The model under review builds one solid part; all positions refer to its coordinate system, in mm. A direction names the side the tool comes from. Round coordinates to 2 decimals unless told otherwise and drop trailing zeros. Write each loop counter-clockwise with the first axis right and the second up, starting at its lowest first coordinate (ties: lowest second). Pieces come first, ordered by that corner, then holes. Notation, with made-up numbers: (0, -33.5) - (20, -33.5) arc R17 cw to (20, -17.5) - close; hole circle Ø8 at (40, -36). An arc over 180 degrees is marked (long way). Use one line per item in the form item = value.
from build123d import *

# Parameters (mm, degrees)
AUFSATZ_LINEAR_AUSTRAGEN1_DEPTH      = 75
AUFSATZ_LINEAR_AUSTRAGEN1_DEPTH_BACK = 56
SKIZZE1_R                            = 19
M8_TAPPED_HOLE1_D                    = 6.8
M8_TAPPED_HOLE1_DEPTH                = 75
M8_TAPPED_HOLE1_TIP                  = 2.042926105
SKIZZE7_W                            = 3.4
SKIZZE7_H                            = 19
CHAMFER1_SIZE                        = 3
CHAMFER1_SIZE2                       = 1.732050808
CUT_EXTRUDE2_DEPTH                   = 80.668061496
CUT_EXTRUDE2_DEPTH_BACK              = 80.668061496
SKETCH2_W                            = 6.5
SKETCH2_H                            = 6


with BuildPart() as part:
    # Skizze1 → Aufsatz-Linear austragen1 (new, two sides: drawn at the far end of the back side and taken through both)
    with BuildSketch(Plane.XY.offset(-AUFSATZ_LINEAR_AUSTRAGEN1_DEPTH_BACK)):
        Circle(SKIZZE1_R)
    extrude(amount=AUFSATZ_LINEAR_AUSTRAGEN1_DEPTH + AUFSATZ_LINEAR_AUSTRAGEN1_DEPTH_BACK)

    # M8 Tapped Hole1
    with Locations(Plane(origin=(0, 0, -56), x_dir=(-1, 0, 0), z_dir=(0, 0, -1))):
        with Locations((0, 0)):
            Hole(M8_TAPPED_HOLE1_D / 2, depth=M8_TAPPED_HOLE1_DEPTH)
            with Locations((0, 0, -(M8_TAPPED_HOLE1_DEPTH + M8_TAPPED_HOLE1_TIP / 2))):  # 118° drill point
                Cone(0, M8_TAPPED_HOLE1_D / 2, M8_TAPPED_HOLE1_TIP, mode=Mode.SUBTRACT)

    # Skizze7 → Tap Drill for M8 Tap1 (revolve, cut)
    with BuildSketch(Plane(origin=(0, 0, 11), x_dir=(0, 0, 1), z_dir=(0, 1, 0))):
        with Locations((1.7, 9.5)):
            Rectangle(SKIZZE7_W, SKIZZE7_H)
    tap_drill_for_m8_tap1 = revolve(axis=Axis((-6.35, 0, 11), (1, 0, 0)), mode=Mode.SUBTRACT)

    # Spiegeln1: Tap Drill for M8 Tap1 across plane
    add(tap_drill_for_m8_tap1.mirror(Plane(origin=(0, 0, 0), x_dir=(0, 0, 1), z_dir=(1, 0, 0))), mode=Mode.SUBTRACT)

    # Chamfer1
    chamfer1_edges = [part.edges().sort_by_distance(p)[0] for p in [
        (-19, 0, -56),
    ]]
    chamfer1_side = [part.faces().sort_by_distance(p)[0] for p in [
        (-19, 0, -28),
    ]]
    chamfer(chamfer1_edges, length=CHAMFER1_SIZE, length2=CHAMFER1_SIZE2, reference=chamfer1_side[0])

    # Sketch2 → Cut-Extrude2 (cut, two sides: drawn at the far end of the back side and taken through both)
    with BuildSketch(Plane(origin=(0, 0, 0), x_dir=(1, 0, 0), z_dir=(0, 1, 0)).offset(-CUT_EXTRUDE2_DEPTH_BACK)):
        with Locations((15.75, -66)):
            Rectangle(SKETCH2_W, SKETCH2_H)
    extrude(amount=CUT_EXTRUDE2_DEPTH + CUT_EXTRUDE2_DEPTH_BACK, mode=Mode.SUBTRACT)


solid = part.part
(1) The part is to be moulded in two halves that separate along X. For faces 4 (the conical face through (-2.259, 17.204, -55.854)), 5 (the cylindrical face through (3.14, -1.3, -22.03)), 6 (the cylindrical face through (-9.633, -1.021, 14.243)), say which applies: +X half, -X half, draft (parallel to the pull), parting line (faces both ways), or undercut.
Geometry results:
face_4 = parting line
face_5 = undercut
face_6 = draft
(2) Add section B-B on z = 57. Write out the cut boundary in (x, y), then the cut area to 3 significant figures.
Geometry results:
outline = circle Ø38 at (0, 0)
area = 1,130 mm2
(3) To check wall thickness, follow L1, parallel to Z at x = 14, y = 0; L2, parallel to Z at x = 16.5, y = 4; L3, parallel to Z at x = 13, y = 2. State the ranges of each line that lie inside material, in increasing order.
Geometry results:
L1 = -56 to 7.6, 14.4 to 63, 69 to 75
L2 = -56 to 63, 69 to 75
L3 = -56 to 8.25, 13.75 to 63, 69 to 75
(4) Add section C-C on x = 16. Count the separate pieces of the cut face and the enclosed holes in it, then the cut area to 3 significant figures.
Geometry results:
separate_pieces = 2
enclosed_holes = 1
area = 2,510 mm2
(5) Insertion check: P1, Ø1, axis at y = 1, z = 37.5, coming from the +X side; P2, Ø8, axis at x = -14.5, z = 9.5, coming from the +Y side; P3, Ø1, axis at x = 13.5, y = 12.5, coming from the -Z side. Each pin has a flat end and moves straight along its axis. Give the tip position at first contact, or say it passes through.
Geometry results:
P1 = 18.99
P2 = 15.84
P3 = -54.91
(6) Machinability: for faces 1 (the cylindrical face through (1.828, 2.867, 15.945)), 2 (the flat face through (15, 0, 63)), 3 (the flat face through (4, 0, -56)), which of the approach directions +Z, -Z, +X, -X, +Y, -Y give a long, thin tool a straight path to every point of the face, cutting with its end or side? Answer none if there is none.
Geometry results:
face_1 = -Z
face_2 = +X, +Y, -Y
face_3 = -Z, +X, -X, +Y, -Y
(7) Add section A-A on z = 12.5. Write out the cut boundary in (x, y), then the cut area to 3 significant figures.
Geometry results:
outline = (-18.75, -3.05) arc R19 ccw to (18.75, -3.05) - (1.5, -3.05) arc R3.4 cw to (-1.5, -3.05) - close; (-18.75, 3.05) - (-1.5, 3.05) arc R3.4 cw to (1.5, 3.05) - (18.75, 3.05) arc R19 ccw to start
area = 902 mm2
